from build123d import *

# Parameters (mm, degrees)
EXTRUDE_THIN1_DEPTH                       = 240
FILLET1_R                                 = 3
SKETCH3_W                                 = 35
SKETCH3_H                                 = 300
EXTRUDE2_DEPTH                            = 7.35
SKETCH7_W                                 = 300
SKETCH7_H                                 = 40
EXTRUDE4_DEPTH                            = 7.35
EXTRUDE5_DEPTH                            = 7.35
TAPPED_HOLE_FOR_8_32_HELICOIL_D           = 4.3942
TAPPED_HOLE_FOR_8_32_HELICOIL_CBORE_D     = 5.27558
TAPPED_HOLE_FOR_8_32_HELICOIL_CBORE_DEPTH = 5.08
SKETCH20_W                                = 240
SKETCH20_H                                = 34
EXTRUDE12_DEPTH                           = 1.35
SKETCH21_W                                = 30.65
SKETCH21_H                                = 240
EXTRUDE13_DEPTH                           = 3.35
SKETCH22_W                                = 240
SKETCH22_H                                = 3
EXTRUDE14_DEPTH                           = 3
SKETCH23_W                                = 5
SKETCH23_H                                = 23
EXTRUDE15_DEPTH                           = 240
SKETCH24_R                                = 3.5687
EXTRUDE16_DEPTH                           = 39.65
SKETCH25_W                                = 80
SKETCH25_H                                = 60.65
EXTRUDE17_DEPTH                           = 10
FILLET4_R                                 = 5
SKETCH31_W                                = 50
SKETCH31_H                                = 10.3
EXTRUDE23_DEPTH                           = 41
FILLET5_R                                 = 3


with BuildPart() as part:
    # Sketch1 → Extrude-Thin1 (new body)
    with BuildSketch(Plane.XY):
        Polygon((0, 50.8), (0, 0), (50.8, 0), (50.8, 6.35), (6.35, 6.35), (6.35, 50.8), align=None)
    extrude(amount=-EXTRUDE_THIN1_DEPTH)

    # Fillet1
    fillet1_edges = [part.edges().sort_by_distance(p)[0] for p in [
        (6.35, 6.35, -120),
        (50.8, 6.35, -120),
        (6.35, 50.8, -120),
    ]]
    fillet(fillet1_edges, radius=FILLET1_R)

    # Sketch3 → Extrude2 (cut, through all)
    with BuildSketch(Plane(origin=(0, 6.35, 0), x_dir=(1, 0, 0), z_dir=(0, 1, 0))):
        with Locations((49.5, 95)):
            Rectangle(SKETCH3_W, SKETCH3_H)
    extrude(amount=-EXTRUDE2_DEPTH, mode=Mode.SUBTRACT)

    # Sketch7 → Extrude4 (cut, through all)
    with BuildSketch(Plane(origin=(6.35, 0, 0), x_dir=(0, 0, -1), z_dir=(1, 0, 0))):
        with Locations((145, 54)):
            Rectangle(SKETCH7_W, SKETCH7_H)
    extrude(amount=-EXTRUDE4_DEPTH, mode=Mode.SUBTRACT)

    # Sketch10 → Extrude5 (cut, through all)
    with BuildSketch(Plane(origin=(6.35, 0, 0), x_dir=(0, 0, -1), z_dir=(1, 0, 0))):
        with BuildLine():
            Line((30, 51.5), (210, 51.5))
            Line((210, 51.5), (210, 26.5))
            ThreePointArc((210, 26.5), (208.535533906, 22.964466094), (205, 21.5))
            Line((205, 21.5), (35, 21.5))
            ThreePointArc((35, 21.5), (31.464466094, 22.964466094), (30, 26.5))
            Line((30, 26.5), (30, 51.5))
        make_face()
    extrude(amount=-EXTRUDE5_DEPTH, mode=Mode.SUBTRACT)

    # Tapped Hole for #8-32 Helicoil (through all)
    with Locations(Plane(origin=(6.35, 23, -15), x_dir=(0, 0, 1), z_dir=(1, 0, 0))):
        with Locations((0, 0), (-210, 0)):
            CounterBoreHole(TAPPED_HOLE_FOR_8_32_HELICOIL_D / 2, TAPPED_HOLE_FOR_8_32_HELICOIL_CBORE_D / 2, TAPPED_HOLE_FOR_8_32_HELICOIL_CBORE_DEPTH)

    # Sketch20 → Extrude12 (cut)
    with BuildSketch(Plane.ZY):
        with Locations((-120, 17)):
            Rectangle(SKETCH20_W, SKETCH20_H)
    extrude(amount=-EXTRUDE12_DEPTH, mode=Mode.SUBTRACT)

    # Sketch21 → Extrude13 (cut)
    with BuildSketch(Plane.XZ):
        with Locations((16.675, -120)):
            Rectangle(SKETCH21_W, SKETCH21_H)
    extrude(amount=-EXTRUDE13_DEPTH, mode=Mode.SUBTRACT)

    # Sketch22 → Extrude14 (add)
    with BuildSketch(Plane(origin=(32, 0, 0), x_dir=(0, 0, -1), z_dir=(1, 0, 0))):
        with Locations((120, 4.85)):
            Rectangle(SKETCH22_W, SKETCH22_H)
    extrude(amount=EXTRUDE14_DEPTH)

    # Sketch23 → Extrude15 (add)
    with BuildSketch(Plane.XY):
        with Locations((37.5, -5.15)):
            Rectangle(SKETCH23_W, SKETCH23_H)
    extrude(amount=-EXTRUDE15_DEPTH)

    # Sketch24 → Extrude16 (cut, through all)
    with BuildSketch(Plane(origin=(40, 0, 0), x_dir=(0, 0, -1), z_dir=(1, 0, 0))):
        with Locations((170, -3.15)):
            Circle(SKETCH24_R)
        with Locations((70, -3.15)):
            Circle(SKETCH24_R)
    extrude(amount=-EXTRUDE16_DEPTH, mode=Mode.SUBTRACT)

    # Sketch25 → Extrude17 (cut)
    with BuildSketch(Plane(origin=(40, 0, 0), x_dir=(0, 0, -1), z_dir=(1, 0, 0))):
        with Locations((120, 3.675)):
            Rectangle(SKETCH25_W, SKETCH25_H)
    extrude(amount=-EXTRUDE17_DEPTH, mode=Mode.SUBTRACT)

    # Fillet4
    fillet4_edges = [part.edges().sort_by_distance(p)[0] for p in [
        (30, 4.85, -160),
        (30, 4.85, -80),
    ]]
    fillet(fillet4_edges, radius=FILLET4_R)

    # Sketch31 → Extrude23 (cut, through all)
    with BuildSketch(Plane(origin=(0, 0, 0), x_dir=(0, 0, -1), z_dir=(1, 0, 0))):
        with Locations((25, -11.5)):
            Rectangle(SKETCH31_W, SKETCH31_H)
        with Locations((215, -11.5)):
            Rectangle(SKETCH31_W, SKETCH31_H)
    extrude(amount=EXTRUDE23_DEPTH, mode=Mode.SUBTRACT)

    # Fillet5
    fillet5_edges = [part.edges().sort_by_distance(p)[0] for p in [
        (40, 6.35, -200),
        (40, 6.35, -40),
        (1.35, 3.35, -120),
    ]]
    fillet(fillet5_edges, radius=FILLET5_R)


solid = part.part
Input: part model. Units: mm. Frame: model coordinates. A direction names the side the tool comes from. Give positions to 0.01 mm unless a question says otherwise; leave off trailing zeros. Write each loop counter-clockwise with the first axis right and the second up, starting at its lowest first coordinate (ties: lowest second). Pieces come first, ordered by that corner, then holes. Notation, with made-up numbers: M 61.25,35 L 68.25,35 A7 cw 68.25,39 Z; hole C 43,48.25 d11. An arc over 180 degrees is marked long. Write item = value, one per line. Start each with the question number.
1) Material intervals for line 1 along Y through (x, z) = (4.85, -15); line 2 along Y through (x, z) = (25.5, -164); line 3 along Z through (x, y) = (3, 23), sorted ascending. Write a range as [from, to].
2) First-contact query: pin 1 Ø9 at (x, z) = (23.5, -148.5) entering from -Y; pin 2 Ø12 at (x, y) = (19.5, -7) entering from -Z; pin 3 Ø5.5 at (x, y) = (38.5, -14) entering from +Z; pin 4 Ø5.5 at (x, z) = (3, -83) entering from +Y. Flat tips, straight axial feed; report the tip coordinate or a pass-through.
3) Draft query along Y for faces 4 (the cylindrical face through (37.535, -2.993, -66.435)), 5 (the flat face through (37, -6.35, -215)), 6 (the cylindrical face through (32, 5, -81)). Return one class per face: +Y half, -Y half, draft (parallel to the pull), parting line (faces both ways), or undercut.
4) Cut plane B-B on z = -225. Return the cut outline in (x, y), then the cut area to 3 significant figures.
5) Cut plane D-D on y = 29. Return the cut outline in (x, z), then the cut area to 3 significant figures.
6) Cut plane C-C on x = 33. Return the cut outline in (y, z), then the cut area to 3 significant figures.
7) Cut plane A-A on y = -3.15. Return the cut outline in (x, z), then the cut area to 3 significant figures.
8) Reachability of faces 1 (the flat face through (4, 30, -210)), 2 (the flat face through (6.35, 16, -118)), 3 (the flat face through (37, -16.65, -175)) from +Z, -Z, +X, -X, +Y, -Y: full face, straight path, thin tool, end or side. Return the list, or none.
Solved:
q1.line_1 = [3.35, 20.36], [25.64, 34]
q1.line_2 = [3.35, 6.35]
q1.line_3 = [-240, -227.64], [-222.36, -208.57], [-31.43, -17.64], [-12.36, 0]
q2.pin_1 = 3.35
q2.pin_2 = through
q2.pin_3 = -50
q2.pin_4 = 21.5
q3.face_4 = undercut
q3.face_5 = -Y half
q3.face_6 = draft
q4.outline = M 1.35,6.35 A3 ccw 4.35,3.35 L 35,3.35 L 35,-6.35 L 40,-6.35 L 40,3.35 A3 ccw 37,6.35 L 9.35,6.35 A3 cw 6.35,9.35 L 6.35,20.36 L 1.35,20.36 Z; M 1.35,25.64 L 6.35,25.64 L 6.35,34 L 1.35,34 Z
q4.area = 274 mm2
q5.outline = M 1.35,-240 L 6.35,-240 L 6.35,-210 L 1.35,-210 Z; M 1.35,-30 L 6.35,-30 L 6.35,0 L 1.35,0 Z
q5.area = 300 mm2
q6.outline = M 3.35,-240 L 6.35,-240 L 6.35,-159.58 L 3.35,-159.58 Z; M 3.35,-80.42 L 6.35,-80.42 L 6.35,0 L 3.35,0 Z
q6.area = 483 mm2
q7.outline = M 35,-240 L 40,-240 L 40,-173.57 L 35,-173.57 Z; M 35,-166.43 L 40,-166.43 L 40,-160 L 35,-160 Z; M 35,-80 L 40,-80 L 40,-73.57 L 35,-73.57 Z; M 35,-66.43 L 40,-66.43 L 40,0 L 35,0 Z
q7.area = 729 mm2
q8.face_1 = +X, -X, +Y
q8.face_2 = +Z, -Z, +X, +Y
q8.face_3 = +Z, -Z, +X, -X, -Y
